```python
from build123d import *

# Parameters (mm, degrees)
SKETCH_1_W               = 180
SKETCH_1_H               = 60
EXTRUDE_1_DEPTH          = 4
SKETCH_4_R               = 2
CUT_EXTRUDE_2_DEPTH      = 50
SKETCH_8_R               = 5
CUT_EXTRUDE_6_DEPTH      = 2
SKETCH_9_W               = 60
SKETCH_9_H               = 60
EXTRUDE_2_DEPTH          = 4
SKETCH_10_W              = 60
SKETCH_10_H              = 60
EXTRUDE_3_DEPTH          = 4
CUT_EXTRUDE_7_DEPTH      = 200.609619007
CUT_EXTRUDE_7_DEPTH_BACK = 200.609619007
SKETCH_11_R              = 2.9
FILLET_1_R               = 2.9
FILLET_2_R               = 2.9
FILLET_3_R               = 10


with BuildPart() as part:
    # 草图1 → 凸台-拉伸1 (new body)
    with BuildSketch(Plane.XY):
        Rectangle(SKETCH_1_W, SKETCH_1_H)
    extrude(amount=EXTRUDE_1_DEPTH)

    # 草图4 → 切除-拉伸2 (cut)
    with BuildSketch(Plane.XY.offset(4)):
        with Locations((-70, 20)):
            Circle(SKETCH_4_R)
        with Locations((-70, -20)):
            Circle(SKETCH_4_R)
        with Locations((70, 20)):
            Circle(SKETCH_4_R)
        with Locations((70, -20)):
            Circle(SKETCH_4_R)
    extrude(amount=-CUT_EXTRUDE_2_DEPTH, mode=Mode.SUBTRACT)

    # 草图8 → 切除-拉伸6 (cut)
    with BuildSketch(Plane.XY.offset(4)):
        with Locations((70, 20)):
            Circle(SKETCH_8_R)
        with Locations((-70, 20)):
            Circle(SKETCH_8_R)
        with Locations((-70, -20)):
            Circle(SKETCH_8_R)
        with Locations((70, -20)):
            Circle(SKETCH_8_R)
    extrude(amount=-CUT_EXTRUDE_6_DEPTH, mode=Mode.SUBTRACT)

    # 草图9 → 凸台-拉伸2 (add)
    with BuildSketch(Plane(origin=(90, 0, 0), x_dir=(0, 0, -1), z_dir=(1, 0, 0))):
        with Locations((-30, 0)):
            Rectangle(SKETCH_9_W, SKETCH_9_H)
    extrude(amount=EXTRUDE_2_DEPTH)

    # 草图10 → 凸台-拉伸3 (add)
    with BuildSketch(Plane.ZY.offset(90)):
        with Locations((30, 0)):
            Rectangle(SKETCH_10_W, SKETCH_10_H)
    extrude(amount=EXTRUDE_3_DEPTH)

    # 草图11 → 切除-拉伸7 (cut, two sides: drawn at the far end of the back side and taken through both)
    with BuildSketch(Plane.ZY.offset(94).offset(-CUT_EXTRUDE_7_DEPTH_BACK)):
        with Locations(Location((40, 0, 0), (0, 0, 270))):
            Circle(SKETCH_11_R)
        with BuildLine():
            Line((47.713451316, 9.192533317), (51.441619452, 13.635591088))
            ThreePointArc((51.441619452, 13.635591088), (40, 17.8), (28.558380548, 13.635591088))
            Line((28.558380548, 13.635591088), (32.286548684, 9.192533317))
            ThreePointArc((32.286548684, 9.192533317), (40, 12), (47.713451316, 9.192533317))
        make_face()
    extrude(amount=CUT_EXTRUDE_7_DEPTH + CUT_EXTRUDE_7_DEPTH_BACK, mode=Mode.SUBTRACT)

    # 圆角1
    fillet_1_edges = [part.edges().sort_by_distance(p)[0] for p in [
        (-92, 13.635591088, 51.441619452),
        (-92, 9.192533317, 47.713451316),
        (-92, 13.635591088, 28.558380548),
        (-92, 9.192533317, 32.286548684),
    ]]
    fillet(fillet_1_edges, radius=FILLET_1_R - 0.0001)  # a hair under: the kernel refuses the full size

    # 圆角2
    fillet_2_edges = [part.edges().sort_by_distance(p)[0] for p in [
        (92, 13.635591088, 28.558380548),
        (92, 13.635591088, 51.441619452),
        (92, 9.192533317, 47.713451316),
        (92, 9.192533317, 32.286548684),
    ]]
    fillet(fillet_2_edges, radius=FILLET_2_R - 0.0001)  # a hair under: the kernel refuses the full size

    # 圆角3
    fillet_3_edges = [part.edges().sort_by_distance(p)[0] for p in [
        (92, 30, 60),
        (92, -30, 60),
        (-92, -30, 60),
        (-92, 30, 60),
    ]]
    fillet(fillet_3_edges, radius=FILLET_3_R)


solid = part.part
```
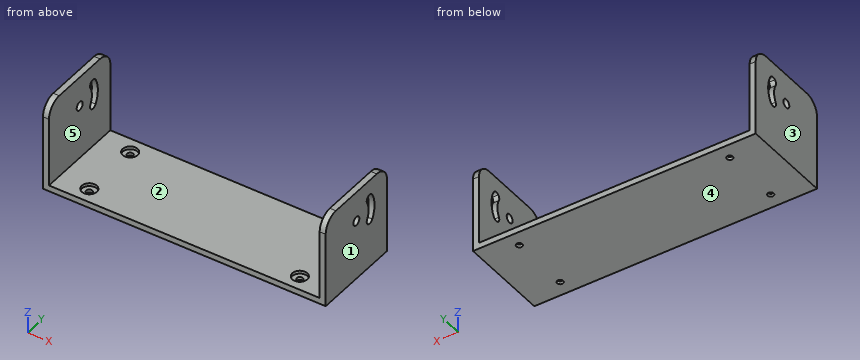
The listing builds one solid part. Answer for the finished solid, in the listing's coordinates (mm). Face numbers are marked on the shaded views. A direction names the side the tool comes from. Round coordinates to 2 decimals unless told otherwise and drop trailing zeros. Loops run counter-clockwise (first coordinate to the right, second up) from the corner with the lowest first, then second, coordinate; pieces in that order, holes last. Notation, with made-up numbers: (84, -15) - (107, -15) arc R21 cw to (107, -8) - close; hole circle Ø5 at (56, -6.5). An arc over 180 degrees is marked (long way). Return JSON: item names as keys, results as strings. Group by question number.
1. Which of the six approach directions +Z, -Z, +X, -X, +Y, -Y give full straight-line access (tool end or side, diameter ignored) to the marked faces 1 and 2?
2. The part is cut by section B-B on y = 0. Determine the outline of the cut face in (x, z), then the cut area to 3 significant figures.
3. Consider probe 1 along Y at (x, z) = (70, 0.5); probe 2 along X at (y, z) = (4.5, 46); probe 3 along Z at (x, y) = (-41, 18.5). Determine where each line is inside the solid, lowest interval first.
4. The part is cut by section C-C on x = -70. Determine the outline of the cut face in (y, z), then the cut area to 3 significant figures.
5. Each of these flat-tipped pins is pushed along its axis until it touches: P1, Ø11, axis at x = -68, y = 18.5, coming from the +Z side; P2, Ø3, axis at x = 68, y = -22.5, coming from the +Z side. Where does it stop, or does it pass through?
6. The part is cut by section D-D on z = 40. Determine the outline of the cut face in (x, y).
7. The part is cut by section A-A on z = 15. Determine the outline of the cut face in (x, y).
8. The mould has two halves that part along X. Classify the marked faces 3, 4 and 5: pulls with the +X half, pulls with the -X half, needs draft (parallel to the pull), parting line crosses it, or undercut.
Resolved:
{
 "1": {"face 1": "+Z, -Z, +X, +Y, -Y", "face 2": "+Z, +Y, -Y"},
 "2": {"outline": "(-94, 0) - (94, 0) - (94, 37.1) - (90, 37.1) - (90, 4) - (-90, 4) - (-90, 37.1) - (-94, 37.1) - close; (-94, 42.9) - (-90, 42.9) - (-90, 60) - (-94, 60) - close; (90, 42.9) - (94, 42.9) - (94, 60) - (90, 60) - close", "area": "1,150 mm²"},
 "3": {"probe 1": "y = -30 to -22, -18 to 18, 22 to 30", "probe 2": "x = -94 to -90, 90 to 94", "probe 3": "z = 0 to 4"},
 "4": {"outline": "(-30, 0) - (-22, 0) - (-22, 2) - (-25, 2) - (-25, 4) - (-30, 4) - close; (-18, 0) - (18, 0) - (18, 2) - (15, 2) - (15, 4) - (-15, 4) - (-15, 2) - (-18, 2) - close; (22, 0) - (30, 0) - (30, 4) - (25, 4) - (25, 2) - (22, 2) - close", "area": "184 mm²"},
 "5": {"P1": "stops at z = 4", "P2": "stops at z = 2"},
 "6": {"outline": "(-94, -30) - (-90, -30) - (-90, -2.9) - (-94, -2.9) - close; (-94, 2.9) - (-90, 2.9) - (-90, 12) - (-94, 12) - close; (-94, 17.8) - (-90, 17.8) - (-90, 30) - (-94, 30) - close; (90, -30) - (94, -30) - (94, -2.9) - (90, -2.9) - close; (90, 2.9) - (94, 2.9) - (94, 12) - (90, 12) - close; (90, 17.8) - (94, 17.8) - (94, 30) - (90, 30) - close"},
 "7": {"outline": "(-94, -30) - (-90, -30) - (-90, 30) - (-94, 30) - close; (90, -30) - (94, -30) - (94, 30) - (90, 30) - close"},
 "8": {"face 3": "pulls with the -X half", "face 4": "needs draft", "face 5": "undercut"}
}
